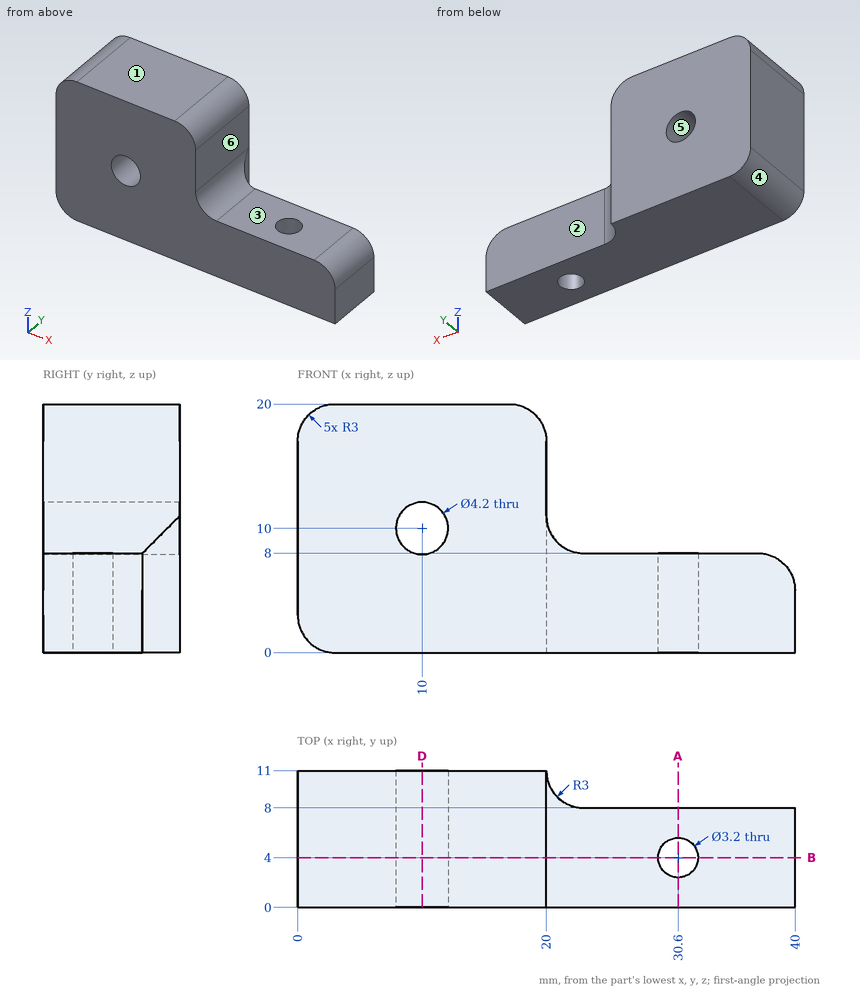
Print and shaded views of the part. All mm, measured from the part's lowest x, y and z. A direction names the side the tool comes from. Coordinates: 2 decimals unless noted, no trailing zeros. Write each loop counter-clockwise with the first axis right and the second up, starting at its lowest first coordinate (ties: lowest second). Pieces come first, ordered by that corner, then holes. Notation, with made-up numbers: (55.25, 3) -> (114.25, 3) arc R23 cw to (114.25, 11) -> close; hole circle Ø1 at (22.5, -36.75). An arc over 180 degrees is marked (long way). Use CSV: the item, a comma, the result in double quotes. Start each with the question number.
Q1. Cut at D-D, the plane x = 10. List the corners of the cut face in (y, z), then the cut area to 3 significant figures.
Q2. Drill centre lines: probe 1 along Y at (x, z) = (30.6, 3); probe 2 along X at (y, z) = (4.25, 13); probe 3 along Z at (x, y) = (27, 5.5). Where is each one in solid material? Low to high.
Q3. Cut at B-B, the plane y = 4. List the corners of the cut face in (x, z), then the cut area to 3 significant figures.
Q4. Cut at A-A, the plane x = 30.6. List the corners of the cut face in (y, z), then the cut area to 3 significant figures.
Q5. 3-axis set-ups, long thin cutter, end or side, ignore diameter. For the marked faces 1, 2 and 3: which of +Z, -Z, +X, -X, +Y, -Y reach the whole face in a straight line?
Q6. Flat gauge pins, fed straight in: pin 1 Ø3.5 at (x, z) = (10, 10) entering from -Y; pin 2 Ø1 at (x, z) = (24.5, 3.5) entering from +Y; pin 3 Ø4 at (x, y) = (32.5, 5.5) entering from +Z; pin 4 Ø6 at (y, z) = (6.5, 12.5) entering from +X. Where does each tip first touch, or does it go through?
Q7. Pull direction Z, two halves, no side cores. Call the marked faces 4, 5 and 6: released by +Z, released by -Z, zero draft, split by the parting line, or undercut.
Checked values:
1,outline,"(0, 0) -> (11, 0) -> (11, 7.9) -> (0, 7.9) -> close; (0, 12.1) -> (11, 12.1) -> (11, 20) -> (0, 20) -> close"
1,area,"174 mm²"
2,probe 1,"y = 0 to 2.4, 5.6 to 8"
2,probe 2,"x = 0 to 20"
2,probe 3,"z = 0 to 8"
3,outline,"(0, 3) arc R3 ccw to (3, 0) -> (29, 0) -> (29, 8) -> (23, 8) arc R3 cw to (20, 11) -> (20, 17) arc R3 ccw to (17, 20) -> (3, 20) arc R3 ccw to (0, 17) -> close; (32.2, 0) -> (40, 0) -> (40, 5) arc R3 ccw to (37, 8) -> (32.2, 8) -> close; hole circle Ø4.2 at (10, 10)"
3,area,"515 mm²"
4,outline,"(0, 0) -> (2.4, 0) -> (2.4, 8) -> (0, 8) -> close; (5.6, 0) -> (8, 0) -> (8, 8) -> (5.6, 8) -> close"
4,area,"38.4 mm²"
5,face 1,"+Z, +X, -X, +Y, -Y"
5,face 2,"+Z, -Z, +X, +Y"
5,face 3,"+Z, +X, +Y, -Y"
6,pin 1,"passes through"
6,pin 2,"stops at y = 8"
6,pin 3,"stops at z = 8"
6,pin 4,"stops at x = 20.4"
7,face 4,"released by -Z"
7,face 5,"undercut"
7,face 6,"zero draft"
